Autodesk Inventor part; units mm, degrees
ref_plane "YZ Plane" through (0, 0, 0) normal (1, 0, 0) x (0, 1, 0)
ref_plane "XZ Plane" through (0, 0, 0) normal (0, 1, 0) x (-1, 0, 0)
ref_plane "XY Plane" through (0, 0, 0) normal (0, 0, 1) x (1, 0, 0)
sketch "Sketch1" plane through (0, 0, 0) normal (0, 0, 1) x (1, 0, 0)
  line L0 (-28, 35.5) -> (28, 35.5)
  line L1 (28, 35.5) -> (28, -35.5)
  line L2 (28, -35.5) -> (-28, -35.5)
  line L3 (-28, -35.5) -> (-28, 35.5)
  line L4 (-20.5, 32.5) -> (23, 32.5)
  line L5 (23, 32.5) -> (23, -30.5)
  line L6 (23, -30.5) -> (-20.5, -30.5)
  line L7 (-20.5, -30.5) -> (-20.5, 32.5)
  point P0 (0, 0)
  dimension "d0" = 56
  dimension "d1" = 28
  dimension "d2" = 71
  dimension "d3" = 35.5
  dimension "d4" = 3
  dimension "d5" = 7.5
  dimension "d7" = 5
  dimension "d8" = 5
extrude "Extrusion1" add sketch "Sketch1" along normal blind 45
sketch "Sketch2" plane through (-28, -35.5, 0) normal (-1, 0, 0) x (0, 0, 1)
  line L0 (37.5, 60.5) -> (12.5, 60.5)
  line L1 (12.5, 60.5) -> (12.5, 10.5)
  line L2 (12.5, 10.5) -> (37.5, 10.5)
  line L3 (37.5, 10.5) -> (37.5, 60.5)
  point P0 (0, 35.5)
  dimension "d11" = 50
  dimension "d12" = 25
  dimension "d13" = 25
  dimension "d14" = 12.5
extrude "Extrusion2" cut sketch "Sketch2" against normal up to surface (7.5 mm away)
sketch "Sketch4" plane through (-28, -35.5, 0) normal (-1, 0, 0) x (0, 0, 1)
  line L0 (40, 64.25) -> (10, 64.25)
  line L1 (10, 64.25) -> (10, 6.75)
  line L2 (10, 6.75) -> (40, 6.75)
  line L3 (40, 6.75) -> (40, 64.25)
  line L4 (0, 0) -> (0, 71)
  point P0 (0, 35.5)
  dimension "d23" = 57.5
  dimension "d24" = 30
  dimension "d25" = 28.75
  dimension "d26" = 10
extrude "Extrusion4" cut sketch "Sketch4" against normal blind 2.5
sketch "Sketch5" plane through (-28, 35.5, 0) normal (0, 1, 0) x (1, 0, 0)
  line L0 (51.75, -40) -> (4.25, -40)
  line L1 (4.25, -40) -> (4.25, -10)
  line L2 (4.25, -10) -> (51.75, -10)
  line L3 (51.75, -10) -> (51.75, -40)
  line L4 (0, 0) -> (56, 0)
  point P0 (28, 0)
  dimension "d29" = 10
  dimension "d30" = 30
  dimension "d31" = 47.5
  dimension "d32" = 23.75
extrude "Extrusion5" cut sketch "Sketch5" against normal blind 2.5
sketch "Sketch6" plane through (-28, 35.5, 0) normal (0, 1, 0) x (1, 0, 0)
  line L0 (48, -37.5) -> (8, -37.5)
  line L1 (8, -37.5) -> (8, -12.5)
  line L2 (8, -12.5) -> (48, -12.5)
  line L3 (48, -12.5) -> (48, -37.5)
  point P0 (28, 0)
  dimension "d35" = 40
  dimension "d36" = 20
  dimension "d37" = 25
  dimension "d38" = 12.5
extrude "Extrusion6" cut sketch "Sketch6" against normal up to surface (3 mm away)
ref_plane "Work Plane1" through (0, 0, 7.5) normal (0, 0, -1) x (-1, 0, 0)
sketch "Sketch8" plane through (0, 0, 7.5) normal (0, 0, -1) x (-1, 0, 0)
  line L0 (-42, 35.5) -> (-28, 35.5)
  line L1 (-28, 35.5) -> (-28, -35.5)
  line L2 (-28, -35.5) -> (-42, -35.5)
  line L3 (-42, -35.5) -> (-42, 35.5)
  line L4 (-28, -35.5) -> (28, -35.5)
  line L5 (28, -35.5) -> (28, -52)
  line L6 (28, -52) -> (-28, -52)
  line L7 (-28, -52) -> (-28, -35.5)
  line L8 (28, 35.5) -> (47, 35.5)
  line L9 (47, 35.5) -> (47, -35.5)
  line L10 (47, -35.5) -> (28, -35.5)
  line L11 (28, -35.5) -> (28, 35.5)
  line L12 (-28, 35.5) -> (28, 35.5)
  line L13 (28, -35.5) -> (-28, -35.5)
  line L14 (-28, -35.5) -> (-28, 35.5)
  line L15 (28, 35.5) -> (28, -35.5)
  point P0 (0, 0)
equation "\"d7\" = d8"
properties part number "sampleHolderEnclosure"
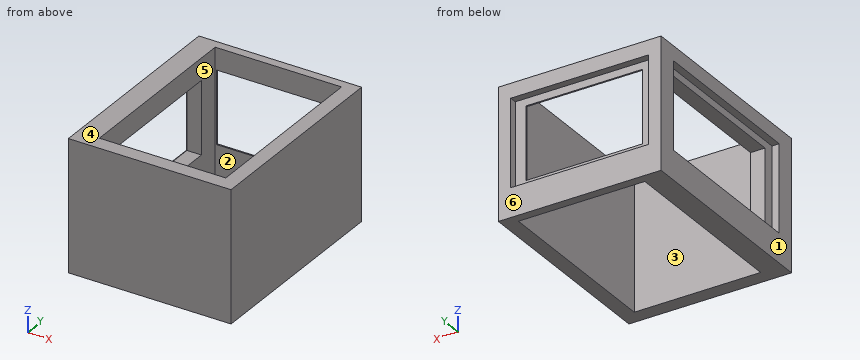
The model under review builds one solid part; all positions refer to its coordinate system, in mm. Face numbers are marked on the shaded views. A direction names the side the tool comes from. Coordinates: 2 decimals unless noted, no trailing zeros. Write each loop counter-clockwise with the first axis right and the second up, starting at its lowest first coordinate (ties: lowest second). Pieces come first, ordered by that corner, then holes. Notation, with made-up numbers: (26, 27) -> (56, 27) arc R14 ccw to (56, 54) -> close; hole circle Ø11 at (-39.5, 8.25). An arc over 180 degrees is marked (long way). One line per item, written item: value. Start each with the question number.
Q1. For the marked faces 5 and 6, list the 3-axis set-ups (+Z, -Z, +X, -X, +Y, -Y) from which the entire face can be reached by the end or side of a thin tool; tool diameter is ignored.
Q2. Add section C-C, the plane y = 30. Give the boundary of the cut face in (x, z), then the cut area to 4 significant figures.
Q3. Add section A-A, the plane z = 36. Give the boundary of the cut face in (x, y).
Q4. Add section D-D, the plane x = -15.5. Give the boundary of the cut face in (y, z).
Q5. To check wall thickness, follow probe 1 along X at (y, z) = (22, 39); probe 2 along X at (y, z) = (-29, 17); probe 3 along Z at (x, y) = (-24, -22). State the ranges of each line that lie inside material, in increasing order.
Q6. Clearance check with flat-ended pins moving along their axes: P1, Ø1.5, axis at y = -26, z = 28, coming from the -X side; P2, Ø2.5, axis at x = -22, z = 23.5, coming from the +Y side; P3, Ø9, axis at y = -6, z = 24.5, coming from the -X side. State where each tip first meets the part, or that it passes through.
Q7. Add section B-B, the plane y = 9.5. Give the boundary of the cut face in (x, z), then the cut area to 4 significant figures.
Q8. The part is to be moulded in two halves that separate along X. For the marked faces 1, 2, 3 and 4, say which applies: +X half, -X half, draft (parallel to the pull), parting line (faces both ways), or undercut.
Response:
1. face 5: +Z, -Z
1. face 6: +Z, -Z, +X, -X, +Y
2. outline: (-28, 0) -> (-20.5, 0) -> (-20.5, 45) -> (-28, 45) -> close; (23, 0) -> (28, 0) -> (28, 45) -> (23, 45) -> close
2. area: 562.5 mm²
3. outline: (-28, -35.5) -> (28, -35.5) -> (28, 35.5) -> (23.75, 35.5) -> (23.75, 33) -> (20, 33) -> (20, 32.5) -> (23, 32.5) -> (23, -30.5) -> (-20.5, -30.5) -> (-20.5, -25) -> (-25.5, -25) -> (-25.5, -28.75) -> (-28, -28.75) -> close; (-28, 28.75) -> (-25.5, 28.75) -> (-25.5, 25) -> (-20.5, 25) -> (-20.5, 32.5) -> (-20, 32.5) -> (-20, 33) -> (-23.75, 33) -> (-23.75, 35.5) -> (-28, 35.5) -> close
4. outline: (-35.5, 0) -> (-30.5, 0) -> (-30.5, 45) -> (-35.5, 45) -> close; (32.5, 0) -> (35.5, 0) -> (35.5, 10) -> (33, 10) -> (33, 12.5) -> (32.5, 12.5) -> close; (32.5, 37.5) -> (33, 37.5) -> (33, 40) -> (35.5, 40) -> (35.5, 45) -> (32.5, 45) -> close
5. probe 1: -25.5 to -20.5, 23 to 28
5. probe 2: -28 to -20.5, 23 to 28
5. probe 3: 0 to 12.5, 37.5 to 45
6. P1: x = -25.5
6. P2: y = 33
6. P3: x = 23
7. outline: (-28, 0) -> (-20.5, 0) -> (-20.5, 12.5) -> (-25.5, 12.5) -> (-25.5, 10) -> (-28, 10) -> close; (-28, 40) -> (-25.5, 40) -> (-25.5, 37.5) -> (-20.5, 37.5) -> (-20.5, 45) -> (-28, 45) -> close; (23, 0) -> (28, 0) -> (28, 45) -> (23, 45) -> close
7. area: 362.5 mm²
8. face 1: -X half
8. face 2: undercut
8. face 3: undercut
8. face 4: draft
